Read the model definition and answer for the solid it produces. Units are mm, in the model's axes. A direction names the side the tool comes from. Coordinates: 2 decimals unless noted, no trailing zeros. Loops run counter-clockwise (first coordinate to the right, second up) from the corner with the lowest first, then second, coordinate; pieces in that order, holes last.
from build123d import *

# Parameters (mm, degrees)
BOSS_EXTRUDE1_DEPTH = 5.08
SKETCH2_R           = 5.08
CUT_EXTRUDE1_DEPTH  = 7.62
CUT_EXTRUDE2_DEPTH  = 7.62


with BuildPart() as part:
    # Sketch1 → Boss-Extrude1 (new body)
    with BuildSketch(Plane(origin=(0, 0, 0), x_dir=(1, 0, 0), z_dir=(0, 1, 0))):
        Polygon((0, 0), (0, 63.5), (50.8, 0), align=None)
    extrude(amount=BOSS_EXTRUDE1_DEPTH)

    # Sketch2 → Cut-Extrude1 (cut)
    with BuildSketch(Plane(origin=(0, 5.08, 0), x_dir=(1, 0, 0), z_dir=(0, 1, 0))):
        with Locations(Location((8.89, 24.13, 0), (0, 0, 270))):
            Circle(SKETCH2_R)
        with Locations(Location((8.89, 38.1, 0), (0, 0, 270))):
            Circle(SKETCH2_R)
        with Locations(Location((16.51, 7.62, 0), (0, 0, 270))):
            Circle(SKETCH2_R)
        with Locations(Location((30.48, 7.62, 0), (0, 0, 270))):
            Circle(SKETCH2_R)
    extrude(amount=-CUT_EXTRUDE1_DEPTH, mode=Mode.SUBTRACT)

    # Sketch3 → Cut-Extrude2 (cut)
    with BuildSketch(Plane(origin=(0, 5.08, 0), x_dir=(1, 0, 0), z_dir=(0, 1, 0))):
        Polygon((18.646117634, 21.012186882), (18.646117634, 40.192352958), (33.990250495, 21.012186882), align=None)
    extrude(amount=-CUT_EXTRUDE2_DEPTH, mode=Mode.SUBTRACT)


solid = part.part
Item 1: A cutting plane is placed at D-D on z = -7.62. Determine the outline of the cut face in (x, y), then the cut area to 3 significant figures.
Numbers:
outline: (0, 0) - (11.43, 0) - (11.43, 5.08) - (0, 5.08) - close; (21.59, 0) - (25.4, 0) - (25.4, 5.08) - (21.59, 5.08) - close; (35.56, 0) - (44.7, 0) - (44.7, 5.08) - (35.56, 5.08) - close
area: 124 mm2
Item 2: A cutting plane is placed at A-A on x = 30.48. Determine the outline of the cut face in (y, z), then the cut area to 3 significant figures.
Numbers:
outline: (0, -21.01) - (5.08, -21.01) - (5.08, -12.7) - (0, -12.7) - close; (0, -2.54) - (5.08, -2.54) - (5.08, 0) - (0, 0) - close
area: 55.1 mm2
Item 3: Determine the mould class of faces 1 (the face through (13.927, 2.576, -38.761)), 2 (the face through (16, 5.08, -22)), 3 (the face through (9.2, 2.5, -52)) for opening direction Z: released by +Z, released by -Z, zero draft, split by the parting line, or undercut.
Numbers:
face 1: undercut
face 2: zero draft
face 3: released by -Z
Item 4: Find the intervals of material crossed by line 1 along Z through (x, y) = (7.5, 2.6) (3 decimals); line 2 along X through (y, z) = (2.4, -7.62); line 3 along X through (y, z) = (0.7, -10.5), in increasing order.
Numbers:
line 1: z = -54.125 to -42.986, -33.214 to -29.016, -19.244 to 0
line 2: x = 0 to 11.43, 21.59 to 25.4, 35.56 to 44.7
line 3: x = 0 to 12.33, 20.69 to 26.3, 34.66 to 42.4
Item 5: Which of the six approach directions +Z, -Z, +X, -X, +Y, -Y give full straight-line access (tool end or side, diameter ignored) to faces 4 (the face through (10.416, 2.576, -19.285)), 5 (the face through (18.646, 3, -30))?
Numbers:
face 4: +Y, -Y
face 5: -Z, +X, +Y, -Y
Item 6: A cutting plane is placed at C-C on z = -24.13. Determine the outline of the cut face in (x, y).
Numbers:
outline: (0, 0) - (3.81, 0) - (3.81, 5.08) - (0, 5.08) - close; (13.97, 0) - (18.65, 0) - (18.65, 5.08) - (13.97, 5.08) - close
Item 7: A cutting plane is placed at B-B on y = 2.35. Determine the outline of the cut face in (x, z).
Numbers:
outline: (0, -63.5) - (18.65, -40.19) - (18.65, -21.01) - (33.99, -21.01) - (50.8, 0) - (0, 0) - close; hole circle Ø10.16 at (8.89, -38.1); hole circle Ø10.16 at (8.89, -24.13); hole circle Ø10.16 at (16.51, -7.62); hole circle Ø10.16 at (30.48, -7.62)
Item 8: Given pin 1 (2.5 mm diameter, centred on y = 3.5, z = -33, fed in from +X); pin 2 (1 mm diameter, centred on y = 2, z = -56.5, fed in from +X); pin 3 (1 mm diameter, centred on x = 24.5, y = 1.5, fed in from -Z), each flat-ended and moving along its own axis, determine where each tip first touches the part or whether it passes through.
Numbers:
pin 1: stops at x = 18.65
pin 2: stops at x = 6
pin 3: stops at z = -21.01
